The model under review builds one solid part; all positions refer to its coordinate system, in mm. Face numbers are marked on the shaded views. A direction names the side the tool comes from. Coordinates: 2 decimals unless noted, no trailing zeros. Loops run counter-clockwise (first coordinate to the right, second up) from the corner with the lowest first, then second, coordinate; pieces in that order, holes last. Notation, with made-up numbers: M -28.75,25.5 L 17.25,25.5 A9 cw 17.25,36.5 Z; hole C 60,34 d10. An arc over 180 degrees is marked long. Use one line per item in the form item = value.
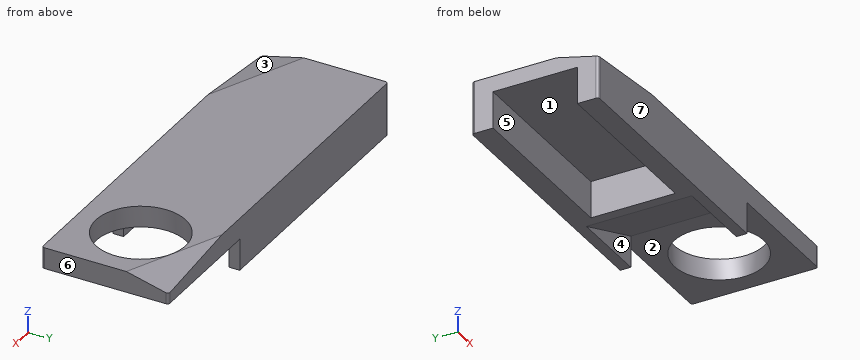
```python
from build123d import *

# Parameters (mm, degrees)
SKETCH_1_W          = 74
SKETCH_1_H          = 24
EXTRUDE_1_DEPTH     = 10
CHAMFER_START       = 7.716439039
CHAMFER_1_OUTLINE_W = 21
CHAMFER_1_OUTLINE_H = 12
CHAMFER_1_DEPTH     = 3.283560961
SKETCH_2_R          = 8.5
CUT_EXTRUDE_1_DEPTH = 10
SKETCH_3_W          = 24
SKETCH_3_H          = 24
CUT_EXTRUDE_2_DEPTH = 6
CHAMFER_START_2     = -24
CHAMFER_3_OUTLINE_W = 21
CHAMFER_3_OUTLINE_H = 11
CHAMFER_3_DEPTH     = 2.565447114
FILLET_1_R          = 0.5
CUT_EXTRUDE_3_DEPTH = 10
SKETCH_5_W          = 33
SKETCH_5_H          = 16
CUT_EXTRUDE_4_DEPTH = 7


with BuildPart() as part:
    # 草图1 → 凸台-拉伸1 (new body)
    with BuildSketch(Plane.XY):
        with Locations((-37, -12)):
            Rectangle(SKETCH_1_W, SKETCH_1_H)
    extrude(amount=EXTRUDE_1_DEPTH)

    # 倒角1: read off the stored shape, not the designer's step
    # 倒角1 outline → 倒角1 (cut)
    with BuildSketch(Plane(origin=(0, 0, 0), x_dir=(0.994240412860114, -0.02599321340810768, -0.1039728536324305), z_dir=(0.10717276443084896, 0.24113871996940994, 0.9645548798776378)).offset(CHAMFER_START)):
        with Locations((-9.5, -6)):
            Rectangle(CHAMFER_1_OUTLINE_W, CHAMFER_1_OUTLINE_H)
    extrude(amount=CHAMFER_1_DEPTH, mode=Mode.SUBTRACT)

    # 草图2 → 切除-拉伸1 (cut)
    with BuildSketch(Plane(origin=(0, 0, 0), x_dir=(-1, 0, 0), z_dir=(0, 0, -1))):
        with Locations((12, -12)):
            Circle(SKETCH_2_R)
    extrude(amount=-CUT_EXTRUDE_1_DEPTH, mode=Mode.SUBTRACT)

    # 草图3 → 切除-拉伸2 (cut)
    with BuildSketch(Plane(origin=(0, 0, 0), x_dir=(-1, 0, 0), z_dir=(0, 0, -1))):
        with Locations((12, -12)):
            Rectangle(SKETCH_3_W, SKETCH_3_H)
    extrude(amount=-CUT_EXTRUDE_2_DEPTH, mode=Mode.SUBTRACT)

    # 倒角3: read off the stored shape, not the designer's step
    # 倒角3 outline → 倒角3 (cut)
    with BuildSketch(Plane(origin=(0, 0, 0), x_dir=(0.994240412860114, -0.02599321340810768, 0.1039728536324305), z_dir=(0.10717276443084896, 0.24113871996940994, -0.9645548798776378)).offset(CHAMFER_START_2)):
        with Locations((-63.5, 17.5)):
            Rectangle(CHAMFER_3_OUTLINE_W, CHAMFER_3_OUTLINE_H)
    extrude(amount=CHAMFER_3_DEPTH, mode=Mode.SUBTRACT)

    # 圆角1
    fillet_1_edges = [part.edges().sort_by_distance(p)[0] for p in [
        (0, 0, 7),
        (-74, -24, 4),
        (0, -24, 8),
        (-74, 0, 5),
    ]]
    fillet(fillet_1_edges, radius=FILLET_1_R)

    # 草图4 → 切除-拉伸3 (cut, symmetric)
    with BuildSketch(Plane(origin=(0, -12, 0), x_dir=(-1, 0, 0), z_dir=(0, -1, 0))):
        Polygon((24, -6), (39, 0), (24, 0), align=None)
    extrude(amount=CUT_EXTRUDE_3_DEPTH, both=True, mode=Mode.SUBTRACT)

    # 草图5 → 切除-拉伸4 (cut)
    with BuildSketch(Plane(origin=(0, 0, 0), x_dir=(-1, 0, 0), z_dir=(0, 0, -1))):
        with Locations((57.5, -12)):
            Rectangle(SKETCH_5_W, SKETCH_5_H)
    extrude(amount=-CUT_EXTRUDE_4_DEPTH, mode=Mode.SUBTRACT)


solid = part.part
```
1. Add section A-A (y = -12). State the section outline as (x, z) points, then the cut area to 3 significant figures.
Response values:
outline = M -74,7 L -41,7 L -41,0 L -39,0 L -24,6 L -20.5,6 L -20.5,10 L -74,10 Z; M -3.5,6 L 0,6 L 0,10 L -3.5,10 Z
area = 252 mm^2
2. Add section D-D (z = 2). State the section outline as (x, y) points.
Response values:
outline = M -74,-23.5 A0.5 ccw -73.5,-24 L -24,-24 L -24,-22 L -34,-22 L -34,-2 L -24,-2 L -24,0 L -73.5,0 A0.5 ccw -74,-0.5 L -74,-4 L -41,-4 L -41,-20 L -74,-20 Z
3. Add section B-B (x = -12). State the section outline as (y, z) points, then the cut area to 3 significant figures.
Response values:
outline = M -24,6 L -20.5,6 L -20.5,10 L -24,10 Z; M -3.5,6 L 0,6 L 0,9.33 L -2.67,10 L -3.5,10 Z
area = 27.1 mm^2
4. Insertion check: P1, Ø5, axis at x = -57.5, y = -11, coming from the -Z side; P2, Ø10, axis at x = -12, y = -12, coming from the +Z side; P3, Ø2, axis at y = -23, z = 2, coming from the +X side. Each pin has a flat end and moves straight along its axis. Give the tip position at first contact, or say it passes through.
Response values:
P1 = 7
P2 = through
P3 = -24
5. The part is to be moulded in two halves that separate along Y. For the marked faces 5, 6 and 7, say which applies: pulls with the +Y half, pulls with the -Y half, needs draft (parallel to the pull), parting line crosses it, or undercut.
Response values:
face_5 = undercut
face_6 = needs draft
face_7 = pulls with the -Y half
6. Wall thickness on line 1 along Y through (x, z) = (-12, 8.5); line 2 along Y through (x, z) = (-51.5, 3.5); line 3 along Z through (x, y) = (-61.5, -11.5): over which ranges is each line inside the solid? List them lowest first. Write a range as from..to.
Response values:
line_1 = -24..-20.5, -3.5..0
line_2 = -24..-20, -4..0
line_3 = 7..10
7. Machinability: for the marked faces 1, 2, 3 and 4, which of the approach directions +Z, -Z, +X, -X, +Y, -Y give a long, thin tool a straight path to every point of the face, cutting with its end or side? Answer none if there is none.
Response values:
face_1 = -Z, -X
face_2 = -Z, +X, +Y, -Y
face_3 = +Z, -X, -Y
face_4 = -Z, +X
8. Add section C-C (x = -47). State the section outline as (y, z) points, then the cut area to 3 significant figures.
Response values:
outline = M -24,0 L -20,0 L -20,7 L -4,7 L -4,0 L 0,0 L 0,10 L -24,10 Z
area = 128 mm^2
